```python
from build123d import *

# Parameters (mm, degrees)
F3_D = 40


with BuildPart() as f1:
    # F0 (on Front) → F1 (revolve)
    with BuildSketch(Plane.XZ):
        Polygon((50, 25), (0, 25), (-50, 25), (-50, 150), (-53, 150), (-53, 0), (0, 0), (53, 0), (53, 150), (50, 150), align=None)
    revolve(axis=Axis((58.566779, 0, 0), (1, 0, 0)))

    # F3 (through all)
    with Locations(Plane.YZ.offset(53)):
        with Locations((0, 0)):
            Hole(F3_D / 2)


solid = f1.part
```
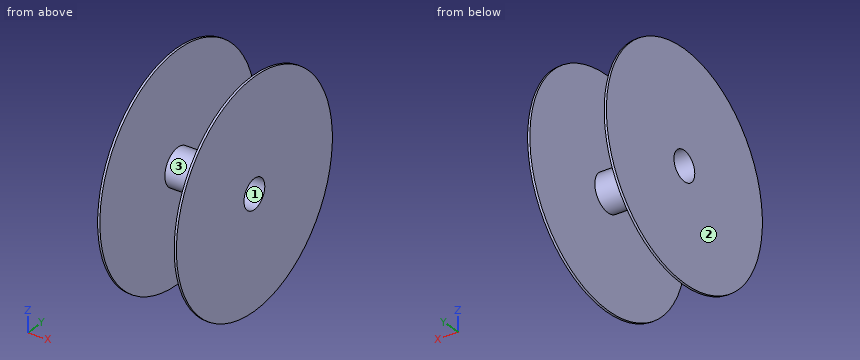
CAD build for the part. Positions are in the model's coordinates, mm. Face numbers are marked on the shaded views. Coordinates: 2 decimals unless noted, no trailing zeros. Order: outer loops, then holes, each group sorted by start corner. A loop starts at its lowest first (then second) coordinate and runs counter-clockwise, first axis right, second up. Notation, with made-up numbers: (67, 24.25) -> (81, 24.25) arc R15 ccw to (81, 39.25) -> close; hole circle Ø5 at (55, 4.5). An arc over 180 degrees is marked (long way). Use one line per item in the form item = value. Start each with the question number.
1) Drop flat-ended pins along their axis: pin 1 (4 mm diameter, centred on x = 18.5, y = -14.5, fed in from -Z); pin 2 (3 mm diameter, centred on x = -13.5, z = 24.5, fed in from +Y). Give the stop position or say it passes through.
2) Drill centre lines: L1, parallel to X at y = -48, z = -50; L2, parallel to Z at x = -22, y = 0; L3, parallel to Y at x = 15.5, z = -0.5 (3 decimals). Where is each one in solid material? Low to high. Write a range as [from, to].
3) Band-saw the part on D-D on y = 94. Give the cut face in (x, z).
4) Band-saw the part on C-C on x = -39. Give the cut face in (y, z), then the cut area to 3 significant figures.
5) Pull direction Y, two halves, no side cores. Call the marked faces 1, 2 and 3: +Y half, -Y half, draft (parallel to the pull), parting line (faces both ways), or undercut.
6) Band-saw the part on A-A on z = 0. Give the cut face in (x, y), then the cut area to 3 significant figures.
Entries:
q1.pin_1 = -21.65
q1.pin_2 = 9.8
q2.L1 = [-53, -50], [50, 53]
q2.L2 = [-25, -20], [20, 25]
q2.L3 = [-24.995, -19.994], [19.994, 24.995]
q3.outline = (-53, -116.89) -> (-50, -116.89) -> (-50, 116.89) -> (-53, 116.89) -> close; (50, -116.89) -> (53, -116.89) -> (53, 116.89) -> (50, 116.89) -> close
q4.outline = circle Ø50 at (0, 0); hole circle Ø40 at (0, 0)
q4.area = 707 mm2
q5.face_1 = undercut
q5.face_2 = draft
q5.face_3 = parting line
q6.outline = (-53, -150) -> (-50, -150) -> (-50, -25) -> (50, -25) -> (50, -150) -> (53, -150) -> (53, -20) -> (-53, -20) -> close; (-53, 20) -> (53, 20) -> (53, 150) -> (50, 150) -> (50, 25) -> (-50, 25) -> (-50, 150) -> (-53, 150) -> close
q6.area = 2,560 mm2
